from build123d import *

# Parameters (mm, degrees)
F0_W     = 79
F0_H     = 55
F1_DEPTH = 23
F2_W     = 75
F2_H     = 51
F3_DEPTH = 16
F4_W     = 12
F4_H     = 4
F5_DEPTH = 55
F6_R     = 3.0875
F7_DEPTH = 25
F8_R     = 5.9215
F9_DEPTH = 1.6


with BuildPart() as f1:
    # F0 (on Front) → F1 (new body)
    with BuildSketch(Plane.XZ):
        Rectangle(F0_W, F0_H)
    extrude(amount=F1_DEPTH)

    # F2 (on face) → F3 (cut)
    with BuildSketch(Plane(origin=(0, 0, 0), x_dir=(-1, 0, 0), z_dir=(0, 1, 0))):
        Rectangle(F2_W, F2_H)
    extrude(amount=-F3_DEPTH, mode=Mode.SUBTRACT)

    # F4 (on Right) → F5 (cut)
    with BuildSketch(Plane.YZ):
        with Locations((-8, 20.5)):
            Rectangle(F4_W, F4_H)
    extrude(amount=F5_DEPTH, mode=Mode.SUBTRACT)

    # F6 (on Front) → F7 (cut)
    with BuildSketch(Plane.XZ):
        with Locations((-11.5, 17.5)):
            Circle(F6_R)
        with Locations((-11.5, 2.5)):
            Circle(F6_R)
        with Locations((3.5, 2.5)):
            Circle(F6_R)
        with Locations((3.5, 17.5)):
            Circle(F6_R)
    extrude(amount=F7_DEPTH, mode=Mode.SUBTRACT)

    # F8 (on face) → F9 (cut)
    with BuildSketch(Plane(origin=(0, -16, 0), x_dir=(-1, 0, 0), z_dir=(0, 1, 0))):
        with Locations((-3.5, 17.5)):
            Circle(F8_R)
        with Locations((-3.5, 2.5)):
            Circle(F8_R)
        with Locations((11.5, 2.5)):
            Circle(F8_R)
        with Locations((11.5, 17.5)):
            Circle(F8_R)
    extrude(amount=-F9_DEPTH, mode=Mode.SUBTRACT)


solid = f1.part
Read the model definition and answer for the solid it produces. Units are mm, in the model's axes. A direction names the side the tool comes from. Coordinates: 2 decimals unless noted, no trailing zeros. Loops run counter-clockwise (first coordinate to the right, second up) from the corner with the lowest first, then second, coordinate; pieces in that order, holes last.
Q1. The part is cut by section A-A on z = 2.5. Write down the section's boundary in (x, y).
Q2. The part is cut by section C-C on y = -20.5. Write down the section's boundary in (x, z) (1 decimal), and give its area (3 significant figures).
Q3. The part is cut by section B-B on x = 3.5. Write down the section's boundary in (y, z).
Q4. Consider probe 1 along X at (y, z) = (-21.75, 2.5); probe 2 along Z at (x, y) = (14, -15.5); probe 3 along X at (y, z) = (-17.25, 3). Determine where each line is inside the solid, lowest interval first.
Q5. Which of the six approach directions +Z, -Z, +X, -X, +Y, -Y give full straight-line access (tool end or side, diameter ignored) to faces 1 (the face through (0.768, -16.789, 12.247)), 2 (the face through (38, -2, 20)), 3 (the face through (4.92, -20.26, -0.24))?
Q6. Each of these flat-tipped pins is pushed along its axis until it touches: pin 1 Ø13 at (x, z) = (-14.5, 18.5) entering from +Y; pin 2 Ø9.5 at (x, z) = (-11.5, 17.5) entering from +Y; pin 3 Ø8 at (x, z) = (-14, 2) entering from -Y. Where does it stop, or does it pass through?
Q7. The mould has two halves that part along Z. Classify faces 4 (the face through (-1, -11, -27.5)), 5 (the face through (1, -8, -25.5)), 6 (the face through (39.5, -11, 0)): +Z half, -Z half, draft (parallel to the pull), parting line (faces both ways), or undercut.
Q8. The part is cut by section D-D on z = -13. Write down the section's boundary in (x, y).
Results below:
1. outline: (-39.5, -23) - (-14.59, -23) - (-14.59, -17.6) - (-17.42, -17.6) - (-17.42, -16) - (-37.5, -16) - (-37.5, 0) - (-39.5, 0) - close; (-8.41, -23) - (0.41, -23) - (0.41, -17.6) - (-2.42, -17.6) - (-2.42, -16) - (-5.58, -16) - (-5.58, -17.6) - (-8.41, -17.6) - close; (6.59, -23) - (39.5, -23) - (39.5, 0) - (37.5, 0) - (37.5, -16) - (9.42, -16) - (9.42, -17.6) - (6.59, -17.6) - close
2. outline: (-39.5, -27.5) - (39.5, -27.5) - (39.5, 27.5) - (-39.5, 27.5) - close; hole circle Ø6.2 at (-11.5, 2.5); hole circle Ø6.2 at (-11.5, 17.5); hole circle Ø6.2 at (3.5, 2.5); hole circle Ø6.2 at (3.5, 17.5)
2. area: 4,230 mm2
3. outline: (-23, -27.5) - (0, -27.5) - (0, -25.5) - (-16, -25.5) - (-16, -3.42) - (-17.6, -3.42) - (-17.6, -0.59) - (-23, -0.59) - close; (-23, 5.59) - (-17.6, 5.59) - (-17.6, 8.42) - (-16, 8.42) - (-16, 11.58) - (-17.6, 11.58) - (-17.6, 14.41) - (-23, 14.41) - close; (-23, 20.59) - (-17.6, 20.59) - (-17.6, 23.42) - (-16, 23.42) - (-16, 25.5) - (0, 25.5) - (0, 27.5) - (-23, 27.5) - close
4. probe 1: x = -39.5 to -14.59, -8.41 to 0.41, 6.59 to 39.5
4. probe 2: z = -27.5 to -25.5, 25.5 to 27.5
4. probe 3: x = -39.5 to -17.4, -5.6 to -2.4, 9.4 to 39.5
5. face 1: +Y
5. face 2: +X
5. face 3: +Y, -Y
6. pin 1: stops at y = -16
6. pin 2: stops at y = -17.6
6. pin 3: stops at y = -23
7. face 4: -Z half
7. face 5: undercut
7. face 6: draft
8. outline: (-39.5, -23) - (39.5, -23) - (39.5, 0) - (37.5, 0) - (37.5, -16) - (-37.5, -16) - (-37.5, 0) - (-39.5, 0) - close
